from build123d import *

# Parameters (mm, degrees)
F1_DEPTH      = 4
F3_DEPTH      = 2.5
F3_DEPTH_BACK = 4


with BuildPart() as f1:
    # F0 (on Top) → F1 (new body)
    with BuildSketch(Plane.XY):
        with BuildLine():
            ThreePointArc((-9.7378284576, 0.4870286754), (-10.3509791066, 0), (-9.7378284576, -0.4870286754))
            ThreePointArc((-9.7378284576, -0.4870286754), (-9.6965884798, -1.0191525169), (-9.6262924975, -1.5482224492))
            ThreePointArc((-9.6262924975, -1.5482224492), (-10.1247853783, -2.1520895677), (-9.4237745868, -2.5009943098))
            ThreePointArc((-9.4237745868, -2.5009943098), (-9.2728010339, -3.0129156952), (-9.0940413632, -3.5158088236))
            ThreePointArc((-9.0940413632, -3.5158088236), (-9.4560899449, -4.2101224943), (-8.6978565462, -4.4056544918))
            ThreePointArc((-8.6978565462, -4.4056544918), (-8.4437476869, -4.875), (-8.1643369833, -5.3297374816))
            ThreePointArc((-8.1643369833, -5.3297374816), (-8.3741180056, -6.0841528656), (-7.5918004377, -6.1177664318))
            ThreePointArc((-7.5918004377, -6.1177664318), (-7.2456620484, -6.524023412), (-6.8778119004, -6.9107310368))
            ThreePointArc((-6.8778119004, -6.9107310368), (-6.926156926, -7.6922765617), (-6.1539462205, -7.5625026225))
            ThreePointArc((-6.1539462205, -7.5625026225), (-5.7309062099, -7.8879156952), (-5.290693434, -8.1896924843))
            ThreePointArc((-5.290693434, -8.1896924843), (-5.1754895533, -8.9642108603), (-4.4471350235, -8.6767211597))
            ThreePointArc((-4.4471350235, -8.6767211597), (-3.96568227, -8.907068212), (-3.472346277, -9.1107250717))
            ThreePointArc((-3.472346277, -9.1107250717), (-3.1986284523, -9.8443661293), (-2.5459626864, -9.4117253466))
            ThreePointArc((-2.5459626864, -9.4117253466), (-2.0271389855, -9.5369391072), (-1.5022409256, -9.6335752554))
            ThreePointArc((-1.5022409256, -9.6335752554), (-1.0819719393, -10.29427536), (-0.5335195629, -9.7353919734))
            ThreePointArc((-0.5335195629, -9.7353919734), (0, -9.75), (0.5335195629, -9.7353919734))
            ThreePointArc((0.5335195629, -9.7353919734), (1.0819719393, -10.29427536), (1.5022409256, -9.6335752554))
            ThreePointArc((1.5022409256, -9.6335752554), (2.0271389855, -9.5369391072), (2.5459626864, -9.4117253466))
            ThreePointArc((2.5459626864, -9.4117253466), (3.1986284523, -9.8443661293), (3.472346277, -9.1107250717))
            ThreePointArc((3.472346277, -9.1107250717), (3.96568227, -8.907068212), (4.4471350235, -8.6767211597))
            ThreePointArc((4.4471350235, -8.6767211597), (5.1754895533, -8.9642108603), (5.290693434, -8.1896924843))
            ThreePointArc((5.290693434, -8.1896924843), (5.7309062099, -7.8879156952), (6.1539462205, -7.5625026225))
            ThreePointArc((6.1539462205, -7.5625026225), (6.926156926, -7.6922765617), (6.8778119004, -6.9107310368))
            ThreePointArc((6.8778119004, -6.9107310368), (7.2456620484, -6.524023412), (7.5918004377, -6.1177664318))
            ThreePointArc((7.5918004377, -6.1177664318), (8.3741180056, -6.0841528656), (8.1643369833, -5.3297374816))
            ThreePointArc((8.1643369833, -5.3297374816), (8.4437476869, -4.875), (8.6978565462, -4.4056544918))
            ThreePointArc((8.6978565462, -4.4056544918), (9.4560899449, -4.2101224943), (9.0940413632, -3.5158088236))
            ThreePointArc((9.0940413632, -3.5158088236), (9.2728010339, -3.0129156952), (9.4237745868, -2.5009943098))
            ThreePointArc((9.4237745868, -2.5009943098), (10.1247853783, -2.1520895677), (9.6262924975, -1.5482224492))
            ThreePointArc((9.6262924975, -1.5482224492), (9.6965884798, -1.0191525169), (9.7378284576, -0.4870286754))
            ThreePointArc((9.7378284576, -0.4870286754), (10.3509791066, 0), (9.7378284576, 0.4870286754))
            ThreePointArc((9.7378284576, 0.4870286754), (9.6965884798, 1.0191525169), (9.6262924975, 1.5482224492))
            ThreePointArc((9.6262924975, 1.5482224492), (10.1247853783, 2.1520895677), (9.4237745868, 2.5009943098))
            ThreePointArc((9.4237745868, 2.5009943098), (9.2728010339, 3.0129156952), (9.0940413632, 3.5158088236))
            ThreePointArc((9.0940413632, 3.5158088236), (9.4560899449, 4.2101224943), (8.6978565462, 4.4056544918))
            ThreePointArc((8.6978565462, 4.4056544918), (8.4437476869, 4.875), (8.1643369833, 5.3297374816))
            ThreePointArc((8.1643369833, 5.3297374816), (8.3741180056, 6.0841528656), (7.5918004377, 6.1177664318))
            ThreePointArc((7.5918004377, 6.1177664318), (7.2456620484, 6.524023412), (6.8778119004, 6.9107310368))
            ThreePointArc((6.8778119004, 6.9107310368), (6.926156926, 7.6922765617), (6.1539462205, 7.5625026225))
            ThreePointArc((6.1539462205, 7.5625026225), (5.7309062099, 7.8879156952), (5.290693434, 8.1896924843))
            ThreePointArc((5.290693434, 8.1896924843), (5.1754895533, 8.9642108603), (4.4471350235, 8.6767211597))
            ThreePointArc((4.4471350235, 8.6767211597), (3.96568227, 8.907068212), (3.472346277, 9.1107250717))
            ThreePointArc((3.472346277, 9.1107250717), (3.1986284523, 9.8443661293), (2.5459626864, 9.4117253466))
            ThreePointArc((2.5459626864, 9.4117253466), (2.0271389855, 9.5369391072), (1.5022409256, 9.6335752554))
            ThreePointArc((1.5022409256, 9.6335752554), (1.0819719393, 10.29427536), (0.5335195629, 9.7353919734))
            ThreePointArc((0.5335195629, 9.7353919734), (0, 9.75), (-0.5335195629, 9.7353919734))
            ThreePointArc((-0.5335195629, 9.7353919734), (-1.0819719393, 10.29427536), (-1.5022409256, 9.6335752554))
            ThreePointArc((-1.5022409256, 9.6335752554), (-2.0271389855, 9.5369391072), (-2.5459626864, 9.4117253466))
            ThreePointArc((-2.5459626864, 9.4117253466), (-3.1986284523, 9.8443661293), (-3.472346277, 9.1107250717))
            ThreePointArc((-3.472346277, 9.1107250717), (-3.96568227, 8.907068212), (-4.4471350235, 8.6767211597))
            ThreePointArc((-4.4471350235, 8.6767211597), (-5.1754895533, 8.9642108603), (-5.290693434, 8.1896924843))
            ThreePointArc((-5.290693434, 8.1896924843), (-5.7309062099, 7.8879156952), (-6.1539462205, 7.5625026225))
            ThreePointArc((-6.1539462205, 7.5625026225), (-6.926156926, 7.6922765617), (-6.8778119004, 6.9107310368))
            ThreePointArc((-6.8778119004, 6.9107310368), (-7.2456620484, 6.524023412), (-7.5918004377, 6.1177664318))
            ThreePointArc((-7.5918004377, 6.1177664318), (-8.3741180056, 6.0841528656), (-8.1643369833, 5.3297374816))
            ThreePointArc((-8.1643369833, 5.3297374816), (-8.4437476869, 4.875), (-8.6978565462, 4.4056544918))
            ThreePointArc((-8.6978565462, 4.4056544918), (-9.4560899449, 4.2101224943), (-9.0940413632, 3.5158088236))
            ThreePointArc((-9.0940413632, 3.5158088236), (-9.2728010339, 3.0129156952), (-9.4237745868, 2.5009943098))
            ThreePointArc((-9.4237745868, 2.5009943098), (-10.1247853783, 2.1520895677), (-9.6262924975, 1.5482224492))
            ThreePointArc((-9.6262924975, 1.5482224492), (-9.6965884798, 1.0191525169), (-9.7378284576, 0.4870286754))
        make_face()
        with BuildLine():
            ThreePointArc((2.5825373774, 1.4258333333), (0, -2.95), (-2.5825373774, 1.4258333333))
            Line((-2.5825373774, 1.4258333333), (-0.7497825806, 1.4258333333))
            Line((-0.7497825806, 1.4258333333), (-0.7497825806, 3.8371907801))
            ThreePointArc((-0.7497825806, 3.8371907801), (-3.7460314761, 2.1114599252), (-4.9297596373, -1.1373001565))
            Line((-4.9297596373, -1.1373001565), (-5.6297596373, -1.1373001565))
            ThreePointArc((-5.6297596373, -1.1373001565), (0.1202403627, 4.6126998435), (5.8702403627, -1.1373001565))
            Line((5.8702403627, -1.1373001565), (5.1702403627, -1.1373001565))
            ThreePointArc((5.1702403627, -1.1373001565), (3.9071710592, 2.2036062924), (0.7497825806, 3.8733062535))
            Line((0.7497825806, 3.8733062535), (0.7497825806, 1.4258333333))
            Line((0.7497825806, 1.4258333333), (2.5825373774, 1.4258333333))
        make_face(mode=Mode.SUBTRACT)
    extrude(amount=F1_DEPTH)

    # F2 (on face) → F3 (join, two sides)
    with BuildSketch(Plane.XY.offset(4)) as f3_sk:
        with BuildLine():
            ThreePointArc((-0.7497825806, 2.8531256688), (-1.8125617033, 2.3274707456), (-2.5825373774, 1.4258333333))
            Line((-2.5825373774, 1.4258333333), (-0.7497825806, 1.4258333333))
            Line((-0.7497825806, 1.4258333333), (-0.7497825806, 2.8531256688))
        make_face()
        with BuildLine():
            Line((0.7497825806, 1.4258333333), (2.5825373774, 1.4258333333))
            ThreePointArc((2.5825373774, 1.4258333333), (1.8125617033, 2.3274707456), (0.7497825806, 2.8531256688))
            Line((0.7497825806, 2.8531256688), (0.7497825806, 1.4258333333))
        make_face()
        with BuildLine():
            ThreePointArc((-0.2497825806, 2.9394061751), (-0.5016410164, 2.9070356535), (-0.7497825806, 2.8531256688))
            Line((-0.7497825806, 2.8531256688), (-0.7497825806, 1.4258333333))
            Line((-0.7497825806, 1.4258333333), (-0.2497825806, 1.4258333333))
            Line((-0.2497825806, 1.4258333333), (-0.2497825806, 2.9394061751))
        make_face()
        with BuildLine():
            Line((0.7497825806, 1.4258333333), (0.7497825806, 2.8531256688))
            ThreePointArc((0.7497825806, 2.8531256688), (0.5016410164, 2.9070356535), (0.2497825806, 2.9394061751))
            Line((0.2497825806, 2.9394061751), (0.2497825806, 1.4258333333))
            Line((0.2497825806, 1.4258333333), (0.7497825806, 1.4258333333))
        make_face()
    extrude(amount=F3_DEPTH)
    extrude(f3_sk.sketch, amount=-F3_DEPTH_BACK)


solid = f1.part
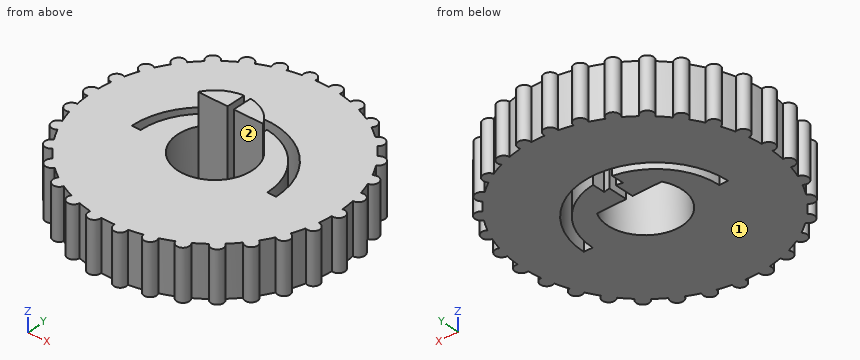
Build history of the part. All positions in model axes, mm. Face numbers are marked on the shaded views. A direction names the side the tool comes from. Give positions to 0.01 mm unless a question says otherwise; leave off trailing zeros. Loops run counter-clockwise (first coordinate to the right, second up) from the corner with the lowest first, then second, coordinate; pieces in that order, holes last. Notation, with made-up numbers: (76, 70) - (91, 70) arc R25 ccw to (91, 90) - close; hole circle Ø2 at (72, 70.5). An arc over 180 degrees is marked (long way). Write item = value, one per line. Start each with the question number.
1) Band-saw the part on A-A on z = 5.25. Give the cut face in (x, y), plus the area to 3 significant figures.
2) Tool access for the marked faces 1 and 2: list every direction of +Z, -Z, +X, -X, +Y, -Y with a clear straight run to the whole face (end or side of a thin tool).
3) Band-saw the part on D-D on y = 3.25. Give the cut face in (x, z).
4) Band-saw the part on B-B on x = 0. Give the cut face in (y, z).
5) Drop flat-ended pins along their axis: pin 1 Ø1.5 at (x, y) = (5, 6) entering from +Z; pin 2 Ø2 at (y, z) = (8, 0.5) entering from +X; pin 3 Ø0.8 at (y, z) = (3.5, 1) entering from -X. Give the stop position or say it passes through.
6) Band-saw the part on C-C on y = 0. Give the cut face in (x, z).
7) Probe probe 1 along Z at (x, y) = (4.5, 5); probe 2 along Y at (x, z) = (-5, 2.5); probe 3 along Y at (x, z) = (3, 0.5). List the from-to ranges inside material, lowest first. Write a range as from..to.
Final values:
q1.outline = (-2.58, 1.43) - (-0.25, 1.43) - (-0.25, 2.94) arc R2.95 ccw to start; (0.25, 1.43) - (2.58, 1.43) arc R2.95 ccw to (0.25, 2.94) - close
q1.area = 4.84 mm²
q2.face_1 = -Z, +X, -X, +Y, -Y
q2.face_2 = +Z, -Z
q3.outline = (-9.19, 0) - (-3.6, 0) - (-3.6, 4) - (-9.19, 4) - close; (-2.38, 0) - (-0.75, 0) - (-0.75, 4) - (-2.38, 4) - close; (0.75, 0) - (2.62, 0) - (2.62, 4) - (0.75, 4) - close; (3.84, 0) - (9.19, 0) - (9.19, 4) - (3.84, 4) - close
q4.outline = (-9.75, 0) - (-2.95, 0) - (-2.95, 4) - (-9.75, 4) - close; (4.61, 0) - (9.75, 0) - (9.75, 4) - (4.61, 4) - close
q5.pin_1 = 4
q5.pin_2 = 7.09
q5.pin_3 = -9.49
q6.outline = (-10.35, 0) - (-5.52, 0) - (-5.52, 4) - (-10.35, 4) - close; (-4.8, 0) - (-2.95, 0) - (-2.95, 4) - (-4.8, 4) - close; (2.95, 0) - (5.04, 0) - (5.04, 4) - (2.95, 4) - close; (5.76, 0) - (10.35, 0) - (10.35, 4) - (5.76, 4) - close
q7.probe_1 = 0..4
q7.probe_2 = -9.03..-1.14, 1.48..9.03
q7.probe_3 = -9.87..3.01, 3.84..9.87
